Geometry check sheet. Reference: drawing and pictorial views, mm from the part's lowest x, y, z. Round coordinates to 2 decimals unless told otherwise and drop trailing zeros. Write each loop counter-clockwise with the first axis right and the second up, starting at its lowest first coordinate (ties: lowest second). Pieces come first, ordered by that corner, then holes. Notation, with made-up numbers: M -34,24 L -7,24 A17 ccw -7,54 Z; hole C -25.75,44 d7. An arc over 180 degrees is marked long. One line per item, written item: value. Start each with the question number.
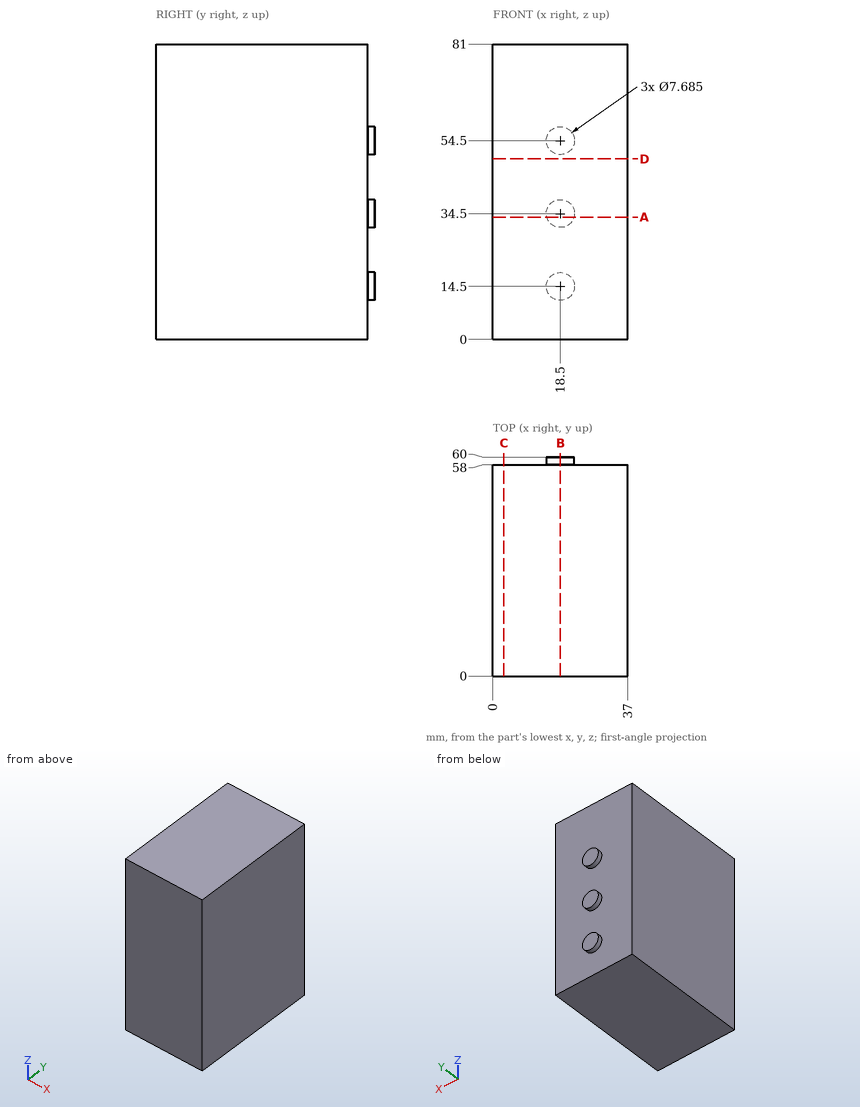
1) Cross-section at D-D (z = 49.5). Record the boundary of the cut face in (x, y), then the cut area to 3 significant figures.
2) Thickness scan on line 1 (Y direction, x = 5, z = 57). Record the ranges inside material, lowest first.
3) Cross-section at A-A (z = 33.5). Record the boundary of the cut face in (x, y), then the cut area to 3 significant figures.
4) Gauge pin test, flat ends, axial feed: pin 1 Ø5 at (x, y) = (10.5, 44) entering from -Z; pin 2 Ø5 at (x, z) = (20.5, 70) entering from +Y. Record the tip position at first contact, or that the pin passes through.
5) Cross-section at B-B (x = 18.5). Record the boundary of the cut face in (y, z), then the cut area to 3 significant figures.
6) Cross-section at C-C (x = 3). Record the boundary of the cut face in (y, z).
Results below:
1. outline: M 0,0 L 37,0 L 37,58 L 0,58 Z
1. area: 2,150 mm²
2. line 1: y = 0 to 58
3. outline: M 0,0 L 37,0 L 37,58 L 22.21,58 L 22.21,60 L 14.79,60 L 14.79,58 L 0,58 Z
3. area: 2,160 mm²
4. pin 1: stops at z = 0
4. pin 2: stops at y = 58
5. outline: M 0,0 L 58,0 L 58,10.66 L 60,10.66 L 60,18.34 L 58,18.34 L 58,30.66 L 60,30.66 L 60,38.34 L 58,38.34 L 58,50.66 L 60,50.66 L 60,58.34 L 58,58.34 L 58,81 L 0,81 Z
5. area: 4,740 mm²
6. outline: M 0,0 L 58,0 L 58,81 L 0,81 Z
